The figure shows three views and two pictorial views of one solid part (mm, origin at its lowest corner). Answer the questions. A direction names the side the tool comes from. Give positions to 0.01 mm unless a question says otherwise; leave off trailing zeros. Write each loop counter-clockwise with the first axis right and the second up, starting at its lowest first coordinate (ties: lowest second). Pieces come first, ordered by that corner, then holes. Notation, with made-up numbers: M -38.5,64 L -10.5,64 A28 cw -10.5,87 Z; hole C 75,88.25 d10. An arc over 180 degrees is marked long. Return JSON: item names as keys, results as strings.
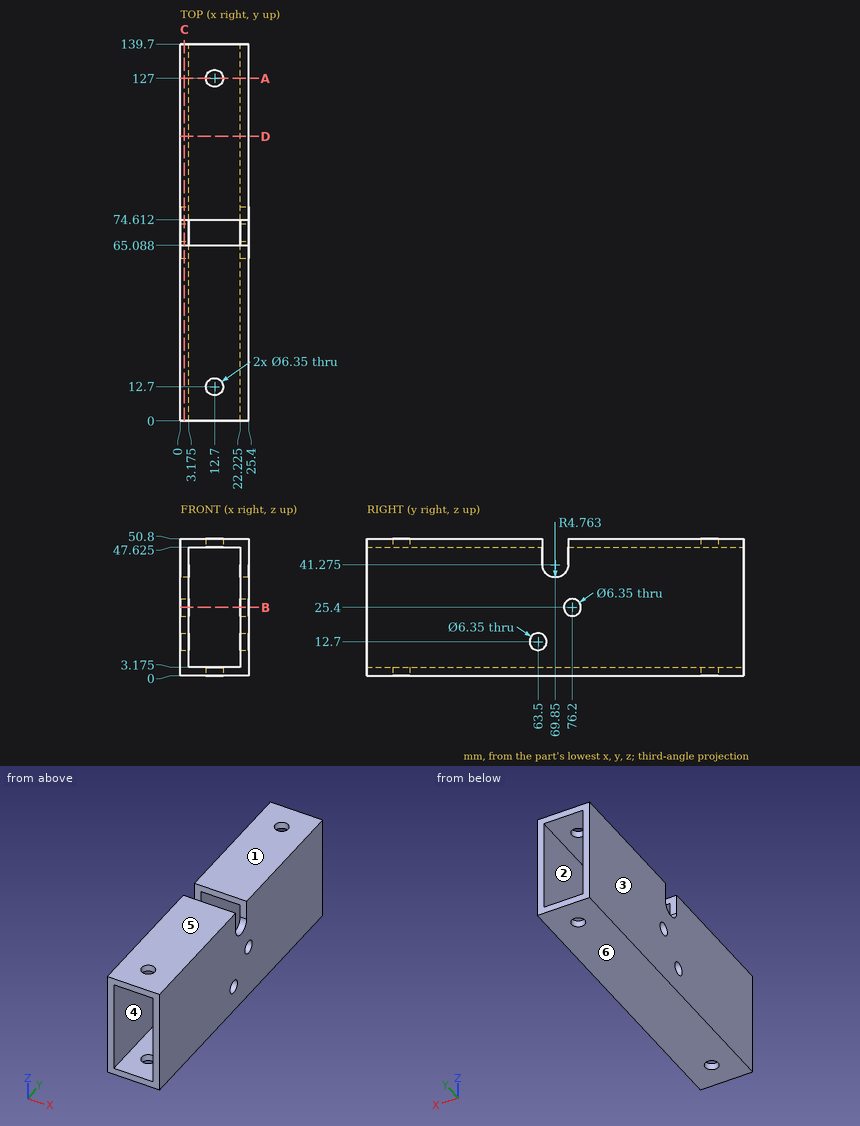
Item 1: Determine the mould class of the marked faces 3, 4, 5 and 6 for opening direction Z: +Z half, -Z half, draft (parallel to the pull), parting line (faces both ways), or undercut.
Geometry results:
{"face 3": "draft", "face 4": "undercut", "face 5": "+Z half", "face 6": "-Z half"}
Item 2: A cutting plane is placed at D-D, the plane y = 105.5. Write down the section's boundary in (x, z) (1 decimal).
Geometry results:
{"outline": "M 0,0 L 25.4,0 L 25.4,50.8 L 0,50.8 Z; hole M 3.2,3.2 L 22.2,3.2 L 22.2,47.6 L 3.2,47.6 Z"}
Item 3: Which of the six approach directions +Z, -Z, +X, -X, +Y, -Y give full straight-line access (tool end or side, diameter ignored) to the marked faces 1 and 2?
Geometry results:
{"face 1": "+Z, +X, -X, +Y, -Y", "face 2": "+Y, -Y"}
Item 4: Find the intervals of material crossed by line 1 (Y direction, x = 12.7, z = 48.6) (1 decimal); line 2 (Z direction, x = 8.5, y = 30) (1 decimal); line 3 (Z direction, x = 23.6, y = 76.2) (1 decimal), in increasing order.
Geometry results:
{"line 1": "y = 0 to 9.5, 15.9 to 65.1, 74.6 to 123.8, 130.2 to 139.7", "line 2": "z = 0 to 3.2, 47.6 to 50.8", "line 3": "z = 0 to 22.2, 28.6 to 50.8"}
Item 5: A cutting plane is placed at A-A, the plane y = 127. Write down the section's boundary in (x, z) (1 decimal).
Geometry results:
{"outline": "M 0,0 L 9.5,0 L 9.5,3.2 L 3.2,3.2 L 3.2,47.6 L 9.5,47.6 L 9.5,50.8 L 0,50.8 Z; M 15.9,0 L 25.4,0 L 25.4,50.8 L 15.9,50.8 L 15.9,47.6 L 22.2,47.6 L 22.2,3.2 L 15.9,3.2 Z"}
Item 6: A cutting plane is placed at C-C, the plane x = 1.5. Count the separate pieces of the cut face and the enclosed holes in it, plus the area to 3 significant figures.
Geometry results:
{"separate pieces": "1", "enclosed holes": "2", "area": "6,910 mm2"}
Item 7: A cutting plane is placed at B-B, the plane z = 25.4. Write down the section's boundary in (x, y) (1 decimal).
Geometry results:
{"outline": "M 0,0 L 3.2,0 L 3.2,73 L 0,73 Z; M 0,79.4 L 3.2,79.4 L 3.2,139.7 L 0,139.7 Z; M 22.2,0 L 25.4,0 L 25.4,73 L 22.2,73 Z; M 22.2,79.4 L 25.4,79.4 L 25.4,139.7 L 22.2,139.7 Z"}
Item 8: Given pin 1 Ø2 at (x, y) = (13.5, 67) entering from +Z (1 decimal); pin 2 Ø5.5 at (x, y) = (12.7, 12.7) entering from +Z, each flat-ended and moving along its own axis, determine where each tip first touches the part or whether it passes through.
Geometry results:
{"pin 1": "stops at z = 3.2", "pin 2": "passes through"}
